from build123d import *

# Parameters (mm, degrees)
SKETCH1_R          = 4.7
EXTRUDE1_DEPTH     = 2
SKETCH2_R          = 4
EXTRUDE2_DEPTH     = 19
SKETCH3_R          = 3
EXTRUDE3_DEPTH     = 5
SKETCH4_R          = 1.5
CUT_EXTRUDE1_DEPTH = 27


with BuildPart() as part:
    # Sketch1 → Extrude1 (new body)
    with BuildSketch(Plane.XY):
        Circle(SKETCH1_R)
    extrude(amount=EXTRUDE1_DEPTH)

    # Sketch2 → Extrude2 (add)
    with BuildSketch(Plane.XY.offset(2)):
        Circle(SKETCH2_R)
    extrude(amount=EXTRUDE2_DEPTH)

    # Sketch3 → Extrude3 (add)
    with BuildSketch(Plane.XY.offset(21)):
        Circle(SKETCH3_R)
    extrude(amount=EXTRUDE3_DEPTH)

    # Sketch4 → Cut-Extrude1 (cut, through all)
    with BuildSketch(Plane(origin=(0, 0, 0), x_dir=(-1, 0, 0), z_dir=(0, 0, -1))):
        Circle(SKETCH4_R)
    extrude(amount=-CUT_EXTRUDE1_DEPTH, mode=Mode.SUBTRACT)


solid = part.part
Part model, mm, in its own coordinate system. A direction names the side the tool comes from. Coordinates: 2 decimals unless noted, no trailing zeros. Order: outer loops, then holes, each group sorted by start corner. A loop starts at its lowest first (then second) coordinate and runs counter-clockwise, first axis right, second up. Notation, with made-up numbers: M -15.5,30 L 31.5,30 A33 ccw 31.5,69 Z; hole C 78,-12 d11. An arc over 180 degrees is marked long. One line per question, with ' | ' between items.
Q1. Slice it at C-C (z = 19.75). Give the cut face in (x, y).
A:
outline: C 0,0 d8; hole C 0,0 d3
Q2. Pin check, flat tips, straight feed: P1, Ø2.5, axis at x = 0, y = 0, coming from the +Z side; P2, Ø3, axis at x = -0.5, z = 13, coming from the +Y side; P3, Ø1.5, axis at x = 3, z = 6, coming from the +Y side; P4, Ø2, axis at x = -0.5, z = 5, coming from the -Y side. Stop position of each tip, or through.
A:
P1: passes through | P2: stops at y = 4 | P3: stops at y = 3.31 | P4: stops at y = -4
Q3. 3-axis set-ups, long thin cutter, end or side, ignore diameter. For faces 1 (the face through (1.3, -1.3, 26)), 2 (the face through (2, 4, 2)): which of +Z, -Z, +X, -X, +Y, -Y reach the whole face in a straight line?
A:
face 1: +Z, +X, -X, +Y, -Y | face 2: +Z
Q4. Slice it at A-A (y = 0). Give the cut face in (x, z).
A:
outline: M -4.7,0 L -1.5,0 L -1.5,26 L -3,26 L -3,21 L -4,21 L -4,2 L -4.7,2 Z; M 1.5,0 L 4.7,0 L 4.7,2 L 4,2 L 4,21 L 3,21 L 3,26 L 1.5,26 Z
Q5. Drill centre lines: line 1 (Y direction, x = 0, z = 20.25); line 2 (Z direction, x = -3.75, y = -2.5); line 3 (X direction, y = -1, z = 15). Where is each one in solid material? Low to high.
A:
line 1: y = -4 to -1.5, 1.5 to 4 | line 2: z = 0 to 2 | line 3: x = -3.87 to -1.12, 1.12 to 3.87
Q6. Two-plate mould, pull along Y, no slides. Class faces 3 (the face through (-3, 0, 23)), 4 (the face through (0, -2, 0)), 5 (the face through (1.5, 0.07, 12.82)): +Y half, -Y half, draft (parallel to the pull), parting line (faces both ways), or undercut.
A:
face 3: parting line | face 4: draft | face 5: undercut
Q7. Slice it at D-D (x = -1.75). Give the cut face in (y, z), and give its area (3 significant figures).
A:
outline: M -4.36,0 L 4.36,0 L 4.36,2 L 3.6,2 L 3.6,21 L 2.44,21 L 2.44,26 L -2.44,26 L -2.44,21 L -3.6,21 L -3.6,2 L -4.36,2 Z | area: 178 mm^2
